Work out the finished part from the listing and answer in its coordinate system (mm). Give positions to 0.01 mm unless a question says otherwise; leave off trailing zeros. Loops run counter-clockwise (first coordinate to the right, second up) from the corner with the lowest first, then second, coordinate; pieces in that order, holes last. Notation, with made-up numbers: (-18, -25.75) - (29, -25.75) arc R27 cw to (29, -5.75) - close; hole circle Ø2 at (22, 41). An arc over 180 degrees is marked (long way). Use one line per item in the form item = value. Start each with the question number.
from build123d import *

# Parameters (mm, degrees)
BOSS_EXTRU_1_DEPTH      = 5
ESQUISSE2_R             = 5
ENL_V_MAT_EXTRU_1_DEPTH = 10


with BuildPart() as part:
    # Esquisse1 → Boss.-Extru.1 (new body)
    with BuildSketch(Plane(origin=(0, 0, 0), x_dir=(1, 0, 0), z_dir=(0, 1, 0))):
        Polygon((0, 0), (50, -86.602540378), (136.602540378, -36.602540378), (136.602540378, 36.602540378), (50, 86.602540378), align=None)
    extrude(amount=BOSS_EXTRU_1_DEPTH)

    # Esquisse2 → Enlèv. mat.-Extru.1 (cut)
    with BuildSketch(Plane(origin=(0, 5, 0), x_dir=(1, 0, 0), z_dir=(0, 1, 0))):
        with Locations(Location((116.602540378, 0, 0), (0, 0, 270))):
            Circle(ESQUISSE2_R)
    extrude(amount=-ENL_V_MAT_EXTRU_1_DEPTH, mode=Mode.SUBTRACT)


solid = part.part
1) A cutting plane is placed at B-B (x = 86). Give the vertices of the cut face in (y, z), plus the area to 3 significant figures.
2) Determine the mould class of faces 1 (the cylindrical face through (121.56, 2.54, -0.65)), 2 (the flat face through (93.91, 2.46, -61.25)), 3 (the flat face through (92.7, 2.46, 61.95)), 4 (the flat face through (67, 0, -1)) for opening direction Z: released by +Z, released by -Z, zero draft, split by the parting line, or undercut.
3) A cutting plane is placed at A-A (y = 3.8). Give the vertices of the cut face in (x, z).
4) A flat-ended cylindrical pin translates along its axis: pin 1 Ø2 at (x, y) = (37, 2) entering from +Z. Find the tip coordinate at first contact, or state that the pin passes through.
5) A cutting plane is placed at C-C (z = 41.5). Give the vertices of the cut face in (x, y).
6) Find the intervals of material crossed by probe 1 along X at (y, z) = (1.45, 0); probe 2 along X at (y, z) = (0.8, 10.5); probe 3 along Z at (x, y) = (111.5, 4.2), in increasing order.
Answer sheet:
q1.outline = (0, -65.82) - (5, -65.82) - (5, 65.82) - (0, 65.82) - close
q1.area = 658 mm²
q2.face_1 = undercut
q2.face_2 = released by -Z
q2.face_3 = released by +Z
q2.face_4 = zero draft
q3.outline = (0, 0) - (50, -86.6) - (136.6, -36.6) - (136.6, 36.6) - (50, 86.6) - close; hole circle Ø10 at (116.6, 0)
q4.pin_1 = 65.82
q5.outline = (23.96, 0) - (128.12, 0) - (128.12, 5) - (23.96, 5) - close
q6.probe_1 = 0 to 111.6, 121.6 to 136.6
q6.probe_2 = 6.06 to 136.6
q6.probe_3 = -51.1 to 51.1
